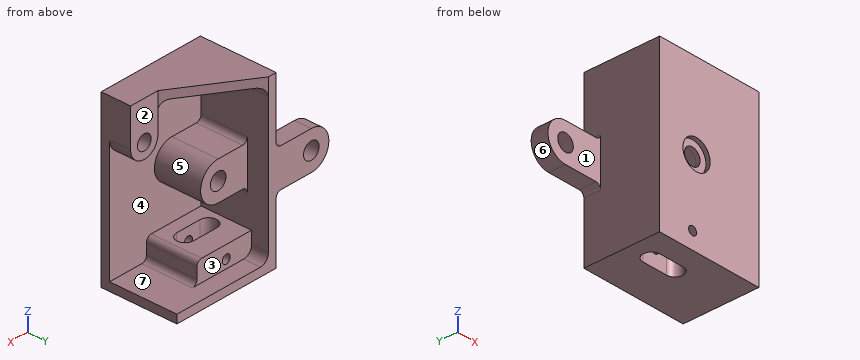
```python
from build123d import *

# Parameters (mm, degrees)
BOSS_EXTRUDE1_DEPTH = 6.35
BOSS_EXTRUDE2_DEPTH = 57.15
FILLET1_R           = 6.35
SKETCH3_R           = 5.6007
BOSS_EXTRUDE3_DEPTH = 22.225
SKETCH4_W           = 127
SKETCH4_H           = 6.35
BOSS_EXTRUDE4_DEPTH = 80.899
BOSS_EXTRUDE5_DEPTH = 38.1
FILLET2_R           = 3.81
SKETCH6_R           = 6.35
BOSS_EXTRUDE6_DEPTH = 34.925
SKETCH7_R           = 6.35
CUT_EXTRUDE1_DEPTH  = 34.925
SKETCH8_R           = 11.1125
CUT_EXTRUDE2_DEPTH  = 3.175
FILLET3_R           = 6.35
SKETCH10_R          = 6.35
BOSS_EXTRUDE7_DEPTH = 12.7
FILLET4_R           = 3.81
CUT_EXTRUDE3_REACH  = 46.45
SKETCH11_R          = 3.241727166
CUT_EXTRUDE4_REACH  = 129


with BuildPart() as part:
    # Sketch1 → Boss-Extrude1 (new body)
    with BuildSketch(Plane.XY):
        Polygon((-25.588082164, 20.346341683), (-31.938082164, 20.346341683), (-31.938082164, -36.803658317), (48.960917836, -36.803658317), (48.960917836, -14.578658317), (26.735917836, -14.578658317), align=None)
    extrude(amount=-BOSS_EXTRUDE1_DEPTH)

    # Sketch2 → Boss-Extrude2 (add)
    with BuildSketch(Plane(origin=(0, 20.346341683, 0), x_dir=(1, 0, 0), z_dir=(0, 1, 0))):
        Polygon((48.960917836, 127), (48.960917836, 120.65), (-25.588082164, 120.65), (-25.588082164, 6.35), (-31.938082164, 6.35), (-31.938082164, 127), (-25.588082164, 127), align=None)
    extrude(amount=-BOSS_EXTRUDE2_DEPTH)

    # Fillet1
    fillet1_edges = [part.edges().sort_by_distance(p)[0] for p in [
        (-25.588082164, -8.228658317, -120.65),
        (-25.588082164, -8.228658317, -6.35),
    ]]
    fillet(fillet1_edges, radius=FILLET1_R)

    # Sketch3 → Boss-Extrude3 (add)
    with BuildSketch(Plane(origin=(0, -14.578658317, 0), x_dir=(1, 0, 0), z_dir=(0, 1, 0))):
        with BuildLine():
            Line((26.735917836, 6.35), (48.960917836, 6.35))
            Line((48.960917836, 6.35), (48.960917836, 28.575))
            ThreePointArc((48.960917836, 28.575), (37.848417836, 39.6875), (26.735917836, 28.575))
            Line((26.735917836, 28.575), (26.735917836, 6.35))
        make_face()
        with Locations((37.848417836, 28.575)):
            Circle(SKETCH3_R, mode=Mode.SUBTRACT)
    extrude(amount=-BOSS_EXTRUDE3_DEPTH)

    # Sketch4 → Boss-Extrude4 (add)
    with BuildSketch(Plane(origin=(48.960917836, 0, 0), x_dir=(0, 0, -1), z_dir=(1, 0, 0))):
        with Locations((63.5, -33.628658317)):
            Rectangle(SKETCH4_W, SKETCH4_H)
    extrude(amount=-BOSS_EXTRUDE4_DEPTH)

    # Sketch5 → Boss-Extrude5 (add)
    with BuildSketch(Plane(origin=(0, -30.453658317, 0), x_dir=(1, 0, 0), z_dir=(0, 1, 0))):
        with BuildLine():
            Line((-25.588082164, 104.775), (18.861917836, 104.775))
            Line((18.861917836, 104.775), (18.861917836, 120.65))
            Line((18.861917836, 120.65), (-19.238082164, 120.65))
            ThreePointArc((-19.238082164, 120.65), (-23.728210225, 118.790128061), (-25.588082164, 114.3))
            Line((-25.588082164, 114.3), (-25.588082164, 104.775))
        make_face()
    extrude(amount=BOSS_EXTRUDE5_DEPTH)

    # Fillet2
    fillet2_edges = [part.edges().sort_by_distance(p)[0] for p in [
        (18.861917836, -11.403658317, -104.775),
        (18.861917836, -11.403658317, -120.65),
    ]]
    fillet(fillet2_edges, radius=FILLET2_R)

    # Sketch6 → Boss-Extrude6 (add)
    with BuildSketch(Plane(origin=(0, -30.453658317, 0), x_dir=(1, 0, 0), z_dir=(0, 1, 0))):
        with BuildLine():
            Line((-1.839082164, 77.8002), (-25.588082164, 77.8002))
            Line((-25.588082164, 77.8002), (-25.588082164, 49.1998))
            Line((-25.588082164, 49.1998), (-1.839082164, 49.1998))
            ThreePointArc((-1.839082164, 49.1998), (12.461117836, 63.5), (-1.839082164, 77.8002))
        make_face()
        with Locations((-1.839082164, 63.5)):
            Circle(SKETCH6_R, mode=Mode.SUBTRACT)
    extrude(amount=BOSS_EXTRUDE6_DEPTH)

    # Sketch7 → Cut-Extrude1 (cut)
    with BuildSketch(Plane(origin=(0, -30.453658317, 0), x_dir=(1, 0, 0), z_dir=(0, 1, 0))):
        with Locations((-1.839082164, 63.5)):
            Circle(SKETCH7_R)
    extrude(amount=-CUT_EXTRUDE1_DEPTH, mode=Mode.SUBTRACT)

    # Sketch8 → Cut-Extrude2 (cut)
    with BuildSketch(Plane.XZ.offset(36.803658317)):
        with Locations((-1.839082164, -63.5)):
            Circle(SKETCH8_R)
    extrude(amount=-CUT_EXTRUDE2_DEPTH, mode=Mode.SUBTRACT)

    # Fillet3
    fillet3_edges = [part.edges().sort_by_distance(p)[0] for p in [
        (26.735917836, -22.516158317, -6.35),
    ]]
    fillet(fillet3_edges, radius=FILLET3_R)

    # Sketch10 → Boss-Extrude7 (add)
    with BuildSketch(Plane(origin=(0, 20.346341683, 0), x_dir=(1, 0, 0), z_dir=(0, 1, 0))):
        with BuildLine():
            Line((-60.640082164, 49.1998), (-31.938082164, 49.1998))
            Line((-31.938082164, 49.1998), (-31.938082164, 77.8002))
            Line((-31.938082164, 77.8002), (-60.640082164, 77.8002))
            ThreePointArc((-60.640082164, 77.8002), (-74.940282164, 63.5), (-60.640082164, 49.1998))
        make_face()
        with Locations((-60.640082164, 63.5)):
            Circle(SKETCH10_R, mode=Mode.SUBTRACT)
    extrude(amount=-BOSS_EXTRUDE7_DEPTH)

    # Fillet4
    fillet4_edges = [part.edges().sort_by_distance(p)[0] for p in [
        (-25.588082164, -12.991158317, -77.8002),
        (-25.588082164, -12.991158317, -49.1998),
        (-31.938082164, 13.996341683, -77.8002),
        (-31.938082164, 13.996341683, -49.1998),
    ]]
    fillet(fillet4_edges, radius=FILLET4_R)

    # Sketch11 → Cut-Extrude3 (cut, up to next)
    with BuildSketch(Plane(origin=(0, 7.646341683, 0), x_dir=(1, 0, 0), z_dir=(0, 1, 0)), mode=Mode.PRIVATE) as cut_extrude3_sk1:
        with Locations((-5.014082164, 114.3)):
            Circle(SKETCH11_R)
    cut_extrude3_tool1 = extrude(cut_extrude3_sk1.sketch, amount=-CUT_EXTRUDE3_REACH, mode=Mode.PRIVATE) & part.part
    add(cut_extrude3_tool1.solids().sort_by_distance((-5.014082, 7.646342, -114.3))[0], mode=Mode.SUBTRACT)

    # Sketch12 → Cut-Extrude4 (cut, up to next)
    with BuildSketch(Plane(origin=(0, 0, -127), x_dir=(-1, 0, 0), z_dir=(0, 0, -1)), mode=Mode.PRIVATE) as cut_extrude4_sk1:
        with BuildLine():
            Line((-4.510928423, -8.228658317), (14.539060991, -8.228658317))
            ThreePointArc((14.539060991, -8.228658317), (20.889071577, -14.578653023), (14.539071577, -20.928658317))
            Line((14.539071577, -20.928658317), (-4.510907248, -20.928658317))
            ThreePointArc((-4.510907248, -20.928658317), (-10.860928423, -14.578668904), (-4.510928423, -8.228658317))
        make_face()
    cut_extrude4_tool1 = extrude(cut_extrude4_sk1.sketch, amount=-CUT_EXTRUDE4_REACH, mode=Mode.PRIVATE) & part.part
    add(cut_extrude4_tool1.solids().sort_by_distance((-5.014072, -14.578658, -127))[0], mode=Mode.SUBTRACT)


solid = part.part
```
The model under review builds one solid part; all positions refer to its coordinate system, in mm. Face numbers are marked on the shaded views. A direction names the side the tool comes from. Round coordinates to 2 decimals unless told otherwise and drop trailing zeros. Loops run counter-clockwise (first coordinate to the right, second up) from the corner with the lowest first, then second, coordinate; pieces in that order, holes last.
1) The part is to be moulded in two halves that separate along X. For the marked faces 4, 5, 6 and 7, say which applies: pulls with the +X half, pulls with the -X half, needs draft (parallel to the pull), parting line crosses it, or undercut.
Values follow:
face 4: undercut
face 5: pulls with the +X half
face 6: pulls with the -X half
face 7: needs draft
2) Consider section B-B on y = -28.5. Give the number of separate pieces and of enclosed holes in the cut face, then the cut area to 3 significant figures.
Values follow:
separate pieces: 1
enclosed holes: 3
area: 3,910 mm2
3) Clearance check with flat-ended pins moving along their axes: P1, Ø16.5, axis at x = -1.84, z = -63.5, coming from the +Y side; P2, Ø21, axis at x = -5, z = -116, coming from the +Y side; P3, Ø6.5, axis at y = -8, z = -112, coming from the +X side; P4, Ø8.5, axis at x = -5.01, z = -114.3, coming from the +Y side. State where each tip first meets the part, or that it passes through.
Values follow:
P1: stops at y = 4.47
P2: stops at y = 20.35
P3: stops at x = 18.86
P4: stops at y = 7.65
4) Consider section C-C on x = 2. State the section outline as (y, z) points (3 decimals).
Values follow:
outline: (-36.804, -127) - (-20.929, -127) - (-20.929, -104.775) - (-30.454, -104.775) - (-30.454, -77.275) - (4.471, -77.275) - (4.471, -68.558) - (-33.629, -68.558) - (-33.629, -73.928) - (-36.804, -73.928) - close; (-36.804, -53.072) - (-33.629, -53.072) - (-33.629, -58.442) - (4.471, -58.442) - (4.471, -49.725) - (-30.454, -49.725) - (-30.454, -6.35) - (1.932, -6.35) - (1.932, 0) - (-36.804, 0) - close; (-8.229, -127) - (20.346, -127) - (20.346, -120.65) - (7.646, -120.65) - (7.646, -104.775) - (-8.229, -104.775) - close
5) Consider section D-D on z = -20.5. State the section outline as (x, y) points, then the cut area to 3 significant figures.
Values follow:
outline: (-31.94, -36.8) - (48.96, -36.8) - (48.96, -14.58) - (26.74, -14.58) - (26.74, -30.45) - (-25.59, -30.45) - (-25.59, 20.35) - (-31.94, 20.35) - close
area: 1,190 mm2
6) Consider section A-A on z = -63.5. State the section outline as (x, y) points.
Values follow:
outline: (-74.94, 7.65) - (-66.99, 7.65) - (-66.99, 20.35) - (-74.94, 20.35) - close; (-54.29, 7.65) - (-31.94, 7.65) - (-31.94, -36.8) - (-12.95, -36.8) - (-12.95, -33.63) - (-8.19, -33.63) - (-8.19, 4.47) - (-25.59, 4.47) - (-25.59, 20.35) - (-54.29, 20.35) - close; (4.51, -33.63) - (9.27, -33.63) - (9.27, -36.8) - (48.96, -36.8) - (48.96, -30.45) - (12.46, -30.45) - (12.46, 4.47) - (4.51, 4.47) - close
7) Wall thickness on line 1 along Y through (x, z) = (0, -107.5); line 2 along X through (y, z) = (-31.75, -63.5); line 3 along X through (y, z) = (11.25, -63.5): over which ranges is each line inside the solid? List them lowest first.
Values follow:
line 1: y = -36.8 to -20.93, -8.23 to 7.65
line 2: x = -31.94 to -8.19, 4.51 to 48.96
line 3: x = -74.94 to -66.99, -54.29 to -25.59
8) Tool access review of the marked faces 1, 2 and 3: name each direction out of +Z, -Z, +X, -X, +Y, -Y from which nothing blocks a thin tool from reaching the whole face with its end or side.
Values follow:
face 1: +Z, -Z, -X, -Y
face 2: +Z, +X, +Y
face 3: +X, +Y
